from build123d import *
from OCP.BRepFilletAPI import BRepFilletAPI_MakeChamfer
from build123d.topology import SkipClean

# Parameters (mm, degrees)
BASPROSKE_W         = 20
BASPROSKE_H         = 16.5
TOOTHCUT_DEPTH      = 31.732718721
TEETHCUTS_COUNT     = 20
TEETHCUTS_ANGLE     = 342
BORSKE_R            = 0.5
BORE_DEPTH          = 50.0000508
BOSS_EXTRUDE1_START = 10
SKETCH1_R           = 7
SKETCH1_R_2         = 0.5
BOSS_EXTRUDE1_DEPTH = 10
FILLET1_R           = 5
SKETCH2_R           = 9
BOSS_EXTRUDE2_DEPTH = 10
SKETCH3_R           = 3
BOSS_EXTRUDE3_DEPTH = 3.2
FILLET2_R           = 4
CUT_EXTRUDE1_DEPTH  = 25
CHAMFER2_SIZE       = 1
CHAMFER2_SIZE2      = 0.176326981
SKETCH5_R           = 2.15
CUT_EXTRUDE2_DEPTH  = 3


with BuildPart() as part:
    # BasProSke → Base-Revolve (revolve)
    with BuildSketch(Plane(origin=(0, 0, 0), x_dir=(1, 0, 0), z_dir=(0, 1, 0)), mode=Mode.PRIVATE) as base_revolve_sk:
        with Locations((10, 8.25)):
            Rectangle(BASPROSKE_W, BASPROSKE_H)
    revolve(base_revolve_sk.sketch.rotate(Axis((-10, 0, 0), (1, 0, 0)), 180), axis=Axis((-10, 0, 0), (1, 0, 0)))

    # TooCutSke → ToothCut (cut, through all)
    with BuildSketch(Plane(origin=(0, 0, 0), x_dir=(0, 0, -1), z_dir=(1, 0, 0))):
        with BuildLine():
            ThreePointArc((0.74381438, 13.102904875), (0, 13.124), (-0.74381438, 13.102904875))
            ThreePointArc((-0.74381438, 13.102904875), (-1.226473103, 14.852072512), (-2.209965745, 16.376962373))
            ThreePointArc((-2.209965745, 16.376962373), (0, 16.5254), (2.209965745, 16.376962373))
            ThreePointArc((2.209965745, 16.376962373), (1.226473103, 14.852072512), (0.74381438, 13.102904875))
        make_face()
    toothcut = extrude(amount=TOOTHCUT_DEPTH, mode=Mode.SUBTRACT)

    # TeethCuts: ToothCut ×20 about axis
    teethcuts_axis = Axis((-10, 0, 0), (1, 0, 0))
    for i in range(1, TEETHCUTS_COUNT):
        add(toothcut.rotate(teethcuts_axis, i * TEETHCUTS_ANGLE / (TEETHCUTS_COUNT - 1)), mode=Mode.SUBTRACT)

    # BorSke → Bore (cut, symmetric)
    with BuildSketch(Plane(origin=(0, 0, 0), x_dir=(0, 0, -1), z_dir=(1, 0, 0))):
        with Locations(Location((0, 0, 0), (0, 0, 180))):
            Circle(BORSKE_R)
    extrude(amount=BORE_DEPTH, both=True, mode=Mode.SUBTRACT)

    # Sketch1 → Boss-Extrude1 (add)
    with BuildSketch(Plane(origin=(20, 0, 0), x_dir=(0, 0, -1), z_dir=(1, 0, 0)).offset(BOSS_EXTRUDE1_START)):
        with Locations(Location((0, 0, 0), (0, 0, 180))):
            Circle(SKETCH1_R)
        Circle(SKETCH1_R_2, mode=Mode.SUBTRACT)
    extrude(amount=-BOSS_EXTRUDE1_DEPTH)

    # Fillet1
    fillet1_edges = [part.edges().sort_by_distance(p)[0] for p in [
        (20, 0, -7),
    ]]
    fillet(fillet1_edges, radius=FILLET1_R)

    # Sketch2 → Boss-Extrude2 (add)
    with BuildSketch(Plane.ZY):
        with Locations(Location((0, 0, 0), (0, 0, 180))):
            Circle(SKETCH2_R)
    extrude(amount=BOSS_EXTRUDE2_DEPTH)

    # Sketch3 → Boss-Extrude3 (add)
    with BuildSketch(Plane.ZY.offset(10)):
        with Locations(Location((0, 0, 0), (0, 0, 270))):
            Circle(SKETCH3_R)
    extrude(amount=BOSS_EXTRUDE3_DEPTH)

    # Fillet2
    fillet2_edges = [part.edges().sort_by_distance(p)[0] for p in [
        (0, 0, 9),
    ]]
    fillet(fillet2_edges, radius=FILLET2_R)

    # Sketch4 → Cut-Extrude1 (cut)
    with BuildSketch(Plane(origin=(30, 0, 0), x_dir=(0, 0, -1), z_dir=(1, 0, 0))):
        with BuildLine():
            Line((-1.378404875, 1.65), (1.378404875, 1.65))
            ThreePointArc((1.378404875, 1.65), (0, -2.15), (-1.378404875, 1.65))
        make_face()
    extrude(amount=-CUT_EXTRUDE1_DEPTH, mode=Mode.SUBTRACT)

    # Chamfer2: one chamfer whose edges measure the first distance from different faces: ONE call of the kernel's chamfer builder (chamfer() names one face for all edges)
    chamfer2_edges_1 = [part.edges().sort_by_distance(p)[0] for p in [
        (30, 1.65, 0),
    ]]
    chamfer2_side_1 = [part.faces().sort_by_distance(p)[0] for p in [
        (17.5, 1.65, 0),
    ]]
    chamfer2_edges_2 = [part.edges().sort_by_distance(p)[0] for p in [
        (30, -2.15, 0),
    ]]
    chamfer2_side_2 = [part.faces().sort_by_distance(p)[0] for p in [
        (17.5, -2.15, 0),
    ]]
    chamfer2 = BRepFilletAPI_MakeChamfer(part.part.solid().wrapped)
    for e in chamfer2_edges_1:
        chamfer2.Add(CHAMFER2_SIZE, CHAMFER2_SIZE2, e.wrapped, chamfer2_side_1[0].wrapped)  # the first distance lies on this face
    for e in chamfer2_edges_2:
        chamfer2.Add(CHAMFER2_SIZE, CHAMFER2_SIZE2, e.wrapped, chamfer2_side_2[0].wrapped)  # the first distance lies on this face
    add(Compound.cast(chamfer2.Shape()), mode=Mode.REPLACE)

    # Sketch5 → Cut-Extrude2 (cut)
    with SkipClean():  # the faces are left unmerged after this step: merging them gives an invalid solid
        with BuildSketch(Plane(origin=(30, 0, 0), x_dir=(0, 0, -1), z_dir=(1, 0, 0))):
            with Locations(Location((0, 0, 0), (0, 0, 50.124722643))):
                Circle(SKETCH5_R)
        extrude(amount=-CUT_EXTRUDE2_DEPTH, mode=Mode.SUBTRACT)


solid = part.part
Check sheet for the modelled part. Datum: model origin and axes. Units: mm. A direction names the side the tool comes from. Round coordinates to 2 decimals unless told otherwise and drop trailing zeros. Loops run counter-clockwise (first coordinate to the right, second up) from the corner with the lowest first, then second, coordinate; pieces in that order, holes last.
1. Mould release check, pull along Z, two halves, no side actions. Record for faces 4 (the cylindrical face through (9.86, 7.723, 10.611)), 5 (the cylindrical face through (9.86, -1.21, 14.815)), 6 (the flat face through (20, 10, -7)), 7 (the cylindrical face through (9.86, -11.274, -9.687)): released by +Z, released by -Z, zero draft, split by the parting line, or undercut.
2. Scan lines: probe 1 along Y at (x, z) = (2.45, 0); probe 2 along Y at (x, z) = (11.5, -13.5); probe 3 along Z at (x, y) = (4, 10.5). Record each from-to range of solid material in increasing order.
3. Set-up check for faces 1 (the cylindrical face through (9.86, -14.815, -1.21)), 2 (the cylindrical face through (9.86, 10.611, -7.723)), 3 (the cylindrical face through (2.535, 0.488, -0.108)): record each of +Z, -Z, +X, -X, +Y, -Y from which the full face is reachable in a straight line by a thin tool's end or side.
4. Sectioned sample at A-A on x = 21. Record the boundary of the cut face in (y, z).
5. Gauge pin test, flat ends, axial feed: pin 1 Ø8 at (x, y) = (19, 8.5) entering from +Z; pin 2 Ø1.1 at (y, z) = (-1, 0.5) entering from +X; pin 3 Ø1 at (y, z) = (-2, -11.5) entering from -X. Record the tip position at first contact, or that the pin passes through.
Recorded:
1. face 4: undercut
1. face 5: released by +Z
1. face 6: zero draft
1. face 7: undercut
2. probe 1: y = -13.12 to -0.5, 0.5 to 13.12
2. probe 2: y = -7.85 to -5.55, -3.45 to -0.8, 0.8 to 3.45, 5.55 to 7.85
2. probe 3: z = -11.67 to -8.64, -7.87 to 7.87, 8.64 to 11.67
3. face 1: +X, -X, -Y
3. face 2: +X, -X
3. face 3: +X
4. outline: circle Ø18 at (0, 0); hole (1.65, -1.38) - (1.65, 1.38) arc R2.15 ccw (long way) to start
5. pin 1: stops at z = 14.88
5. pin 2: stops at x = 5
5. pin 3: stops at x = -0.44
